Read the model definition and answer for the solid it produces. Units are mm, in the model's axes. Round coordinates to 2 decimals unless told otherwise and drop trailing zeros. Loops run counter-clockwise (first coordinate to the right, second up) from the corner with the lowest first, then second, coordinate; pieces in that order, holes last. Notation, with made-up numbers: (-23.75, -26) - (2.25, -26) arc R23 cw to (2.25, 9) - close; hole circle Ø9 at (70, 53). An arc over 180 degrees is marked (long way). Use one line per item in the form item = value. Start each with the question number.
```python
from build123d import *

# Parameters (mm, degrees)
BOSS_EXTRUDE1_DEPTH = 10


with BuildPart() as part:
    # Sketch1 → Boss-Extrude1 (new body)
    with BuildSketch(Plane.XY):
        Polygon((-237.234601608, -129.63585579), (-237.234601608, -87.457773568), (-247.40109201, -87.457773568), (-247.40109201, -3.101609123), (-237.234601608, -3.101609123), (-237.234601608, 81.254555321), (-247.40109201, 81.254555321), (-247.40109201, 165.110720504), (-236.605829759, 165.110720504), (-236.605829759, 175.291552649), (-154.294832327, 175.291552649), (-154.294832327, 165.110720504), (-71.987006932, 165.110720504), (-71.987006932, 175.291552649), (10.110681918, 175.291552649), (10.110681918, 165.110720504), (92.609794057, 165.110720504), (92.609794057, 175.291552649), (174.626730953, 175.291552649), (174.626730953, 165.110720504), (185.669445552, 165.110720504), (185.669445552, 81.254555321), (175.502955151, 81.254555321), (175.502955151, -3.101609123), (185.669445552, -3.101609123), (185.669445552, -87.457773568), (175.502955151, -87.457773568), (175.502955151, -129.63585579), align=None)
        with BuildLine():
            Line((-50.938162507, 125.110720504), (-50.938162507, -5.688963776))
            ThreePointArc((-50.938162507, -5.688963776), (-65.231084294, -24.857408112), (-87.681088334, -16.62854488))
            Line((-87.681088334, -16.62854488), (-173.143675307, 114.1711394))
            ThreePointArc((-173.143675307, 114.1711394), (-173.99040016, 134.629343774), (-156.400749479, 145.110720504))
            Line((-156.400749479, 145.110720504), (-70.938162507, 145.110720504))
            ThreePointArc((-70.938162507, 145.110720504), (-56.796026883, 139.252856128), (-50.938162507, 125.110720504))
        make_face(mode=Mode.SUBTRACT)
        with BuildLine():
            Line((-217.234601608, 41.348661081), (-217.234601608, -89.63585579))
            ThreePointArc((-217.234601608, -89.63585579), (-211.376737232, -103.777991414), (-197.234601608, -109.63585579))
            Line((-197.234601608, -109.63585579), (-111.651247744, -109.63585579))
            ThreePointArc((-111.651247744, -109.63585579), (-94.061597063, -99.15447906), (-94.908321917, -78.696274685))
            Line((-94.908321917, -78.696274685), (-180.491675781, 52.288242186))
            ThreePointArc((-180.491675781, 52.288242186), (-202.941679822, 60.517105417), (-217.234601608, 41.348661081))
        make_face(mode=Mode.SUBTRACT)
        with BuildLine():
            Line((-10.820423043, 125.110720504), (-10.820423043, -5.621130667))
            ThreePointArc((-10.820423043, -5.621130667), (3.47704632, -24.79092838), (25.92769139, -16.552766545))
            Line((25.92769139, -16.552766545), (111.257475845, 114.179084627))
            ThreePointArc((111.257475845, 114.179084627), (112.096753452, 134.633516377), (94.509361412, 145.110720504))
            Line((94.509361412, 145.110720504), (9.179576957, 145.110720504))
            ThreePointArc((9.179576957, 145.110720504), (-4.962558666, 139.252856128), (-10.820423043, 125.110720504))
        make_face(mode=Mode.SUBTRACT)
        with BuildLine():
            Line((118.641820815, 52.310380527), (33.137535964, -78.688818793))
            ThreePointArc((33.137535964, -78.688818793), (32.297563362, -99.141966865), (49.882730912, -109.620454457))
            Line((49.882730912, -109.620454457), (135.387015764, -109.632935879))
            ThreePointArc((135.387015764, -109.632935879), (149.53103864, -103.776103872), (155.389935248, -89.632936092))
            Line((155.389935248, -89.632936092), (155.389935248, 41.37874465))
            ThreePointArc((155.389935248, 41.37874465), (141.092465886, 60.548542362), (118.641820815, 52.310380527))
        make_face(mode=Mode.SUBTRACT)
    extrude(amount=BOSS_EXTRUDE1_DEPTH)


solid = part.part
```
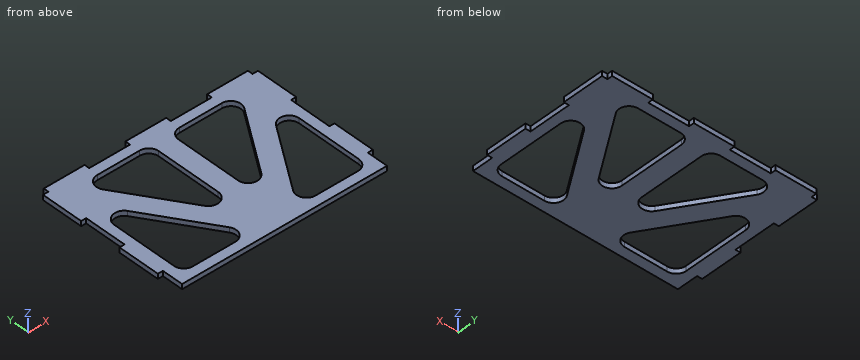
1) Flat-ended cylindrical pins translate along their axes: pin 1 (3 mm diameter, centred on x = -125.5, z = 5.5, fed in from +Y); pin 2 (3 mm diameter, centred on y = 171, z = 5.5, fed in from -X); pin 3 (2 mm diameter, centred on y = 76.5, z = 6.5, fed in from -X). Find the tip coordinate at first contact, or state that the pin passes through.
2) A cutting plane is placed at D-D on y = -11. Write down the section's boundary in (x, z).
3) Straight lines are drawn through the part: line 1 (X direction, y = -91, z = 8.5); line 2 (X direction, y = -26.5, z = 8.5); line 3 (Y direction, x = 98, z = 1.25). For each, find the intervals that lie inside material, in ascending order. Write a range as from..to.
4) A cutting plane is placed at B-B on y = -95. Write down the section's boundary in (x, z), plus the area to 3 significant figures.
5) A cutting plane is placed at C-C on x = -140. Write down the section's boundary in (y, z), plus the area to 3 significant figures.
6) A cutting plane is placed at A-A on x = -79. Write down the section's boundary in (y, z).
Checks:
q1.pin_1 = 165.11
q1.pin_2 = -236.61
q1.pin_3 = -237.23
q2.outline = (-247.4, 0) - (-217.23, 0) - (-217.23, 10) - (-247.4, 10) - close; (-139.14, 0) - (-91.36, 0) - (-91.36, 10) - (-139.14, 10) - close; (-51.66, 0) - (-10.08, 0) - (-10.08, 10) - (-51.66, 10) - close; (29.55, 0) - (77.32, 0) - (77.32, 10) - (29.55, 10) - close; (155.39, 0) - (185.67, 0) - (185.67, 10) - (155.39, 10) - close
q3.line_1 = -237.23..-217.19, -91.7..29.93, 155.34..175.5
q3.line_2 = -247.4..-217.23, -129.01..67.2, 155.39..185.67
q3.line_3 = -129.64..-109.63, 20.69..93.87, 144.8..175.29
q4.outline = (-237.23, 0) - (-216.5, 0) - (-216.5, 10) - (-237.23, 10) - close; (-92.38, 0) - (30.62, 0) - (30.62, 10) - (-92.38, 10) - close; (154.66, 0) - (175.5, 0) - (175.5, 10) - (154.66, 10) - close
q4.area = 1,650 mm²
q5.outline = (-129.64, 0) - (-109.64, 0) - (-109.64, 10) - (-129.64, 10) - close; (-9.68, 0) - (63.45, 0) - (63.45, 10) - (-9.68, 10) - close; (145.11, 0) - (165.11, 0) - (165.11, 10) - (145.11, 10) - close
q5.area = 1,130 mm²
q6.outline = (-129.64, 0) - (-23.99, 0) - (-23.99, 10) - (-129.64, 10) - close; (145.11, 0) - (165.11, 0) - (165.11, 10) - (145.11, 10) - close
